from build123d import *

# Parameters (mm, degrees)
SKETCH1_W           = 94.5
SKETCH1_H           = 70
BOSS_EXTRUDE1_DEPTH = 3
SKETCH3_R           = 1.5
CUT_EXTRUDE2_DEPTH  = 59.877521177
FILLET2_R           = 3
CUT_EXTRUDE3_DEPTH  = 59.877521177
FILLET3_R           = 3


with BuildPart() as part:
    # Sketch1 → Boss-Extrude1 (new body)
    with BuildSketch(Plane(origin=(0, 0, 0), x_dir=(1, 0, 0), z_dir=(0, 1, 0))):
        Rectangle(SKETCH1_W, SKETCH1_H)
    extrude(amount=BOSS_EXTRUDE1_DEPTH)

    # Sketch3 → Cut-Extrude2 (cut, through all)
    with BuildSketch(Plane(origin=(0, 3, 0), x_dir=(1, 0, 0), z_dir=(0, 1, 0))):
        with Locations(Location((43.75, 31.5, 0), (0, 0, 270))):
            Circle(SKETCH3_R)
        with Locations(Location((-43.25, 31.5, 0), (0, 0, 270))):
            Circle(SKETCH3_R)
        with Locations(Location((-43.25, -31.5, 0), (0, 0, 270))):
            Circle(SKETCH3_R)
        with Locations(Location((43.75, -31.5, 0), (0, 0, 270))):
            Circle(SKETCH3_R)
    extrude(amount=-CUT_EXTRUDE2_DEPTH, mode=Mode.SUBTRACT)

    # Fillet2
    fillet2_edges = [part.edges().sort_by_distance(p)[0] for p in [
        (47.25, 1.5, 35),
        (-47.25, 1.5, 35),
        (-47.25, 1.5, -35),
        (47.25, 1.5, -35),
    ]]
    fillet(fillet2_edges, radius=FILLET2_R)

    # Sketch5 → Cut-Extrude3 (cut, through all)
    with BuildSketch(Plane(origin=(0, 3, 0), x_dir=(1, 0, 0), z_dir=(0, 1, 0))):
        Polygon((43.25, 29), (-42.25, 29), (-42.25, 10), (-42.25, -10), (-42.25, -28), (-35, -28), (43.25, -28), align=None)
    extrude(amount=-CUT_EXTRUDE3_DEPTH, mode=Mode.SUBTRACT)

    # Fillet3
    fillet3_edges = [part.edges().sort_by_distance(p)[0] for p in [
        (-42.25, 1.5, 28),
        (-42.25, 1.5, -29),
    ]]
    fillet(fillet3_edges, radius=FILLET3_R)


solid = part.part
Part model, mm, in its own coordinate system. A direction names the side the tool comes from. Round coordinates to 2 decimals unless told otherwise and drop trailing zeros. Write each loop counter-clockwise with the first axis right and the second up, starting at its lowest first coordinate (ties: lowest second). Pieces come first, ordered by that corner, then holes. Notation, with made-up numbers: M -25.5,77 L -3.5,77 A19 ccw -3.5,110 Z; hole C -23,-3.75 d8. An arc over 180 degrees is marked long. Return JSON: item names as keys, results as strings. Group by question number.
(1) Saw through at B-B on y = 1.2. Write the cut outline in (x, z).
(2) Saw through at A-A on z = 10. Write the cut outline in (x, y).
(3) Which spindle directions (+Z, -Z, +X, -X, +Y, -Y) get a long thin tool onto all of the face, cutting with end or side? Do faces 1 (the face through (1, 2, 28)), 2 (the face through (3.3, 0, 28.4)). Say none if no direction does.
(4) Saw through at C-C on x = -43.25. Write the cut outline in (y, z), then the cut area to 3 significant figures.
(5) Saw through at D-D on x = -26.5. Write the cut outline in (y, z), then the cut area to 3 significant figures.
(6) Two-plate mould, pull along Z, no slides. Class faces 3 (the face through (-1, 1, 35)), 4 (the face through (-42.25, 2, -1)), 5 (the face through (-47.25, 1, 0)): +Z half, -Z half, draft (parallel to the pull), parting line (faces both ways), or undercut.
(7) Drill centre lines: probe 1 along X at (y, z) = (1.4, -31.5); probe 2 along X at (y, z) = (2.25, 19); probe 3 along Z at (x, y) = (-8, 1.25). Where is each one in solid material? Low to high.
Returned:
{
 "1": {"outline": "M -47.25,-32 A3 ccw -44.25,-35 L 44.25,-35 A3 ccw 47.25,-32 L 47.25,32 A3 ccw 44.25,35 L -44.25,35 A3 ccw -47.25,32 Z; hole C -43.25,-31.5 d3; hole C -43.25,31.5 d3; hole M -42.25,-26 A3 ccw -39.25,-29 L 43.25,-29 L 43.25,28 L -39.25,28 A3 ccw -42.25,25 Z; hole C 43.75,-31.5 d3; hole C 43.75,31.5 d3"},
 "2": {"outline": "M -47.25,0 L -42.25,0 L -42.25,3 L -47.25,3 Z; M 43.25,0 L 47.25,0 L 47.25,3 L 43.25,3 Z"},
 "3": {"face 1": "+Y, -Y", "face 2": "+Z, -Z, +X, -X, -Y"},
 "4": {"outline": "M 0,-35 L 3,-35 L 3,-33 L 0,-33 Z; M 0,-30 L 3,-30 L 3,30 L 0,30 Z; M 0,33 L 3,33 L 3,35 L 0,35 Z", "area": "192 mm²"},
 "5": {"outline": "M 0,-35 L 3,-35 L 3,-29 L 0,-29 Z; M 0,28 L 3,28 L 3,35 L 0,35 Z", "area": "39.0 mm²"},
 "6": {"face 3": "+Z half", "face 4": "undercut", "face 5": "draft"},
 "7": {"probe 1": "-47.25 to -44.75, -41.75 to 42.25, 45.25 to 47.25", "probe 2": "-47.25 to -42.25, 43.25 to 47.25", "probe 3": "-35 to -29, 28 to 35"}
}
